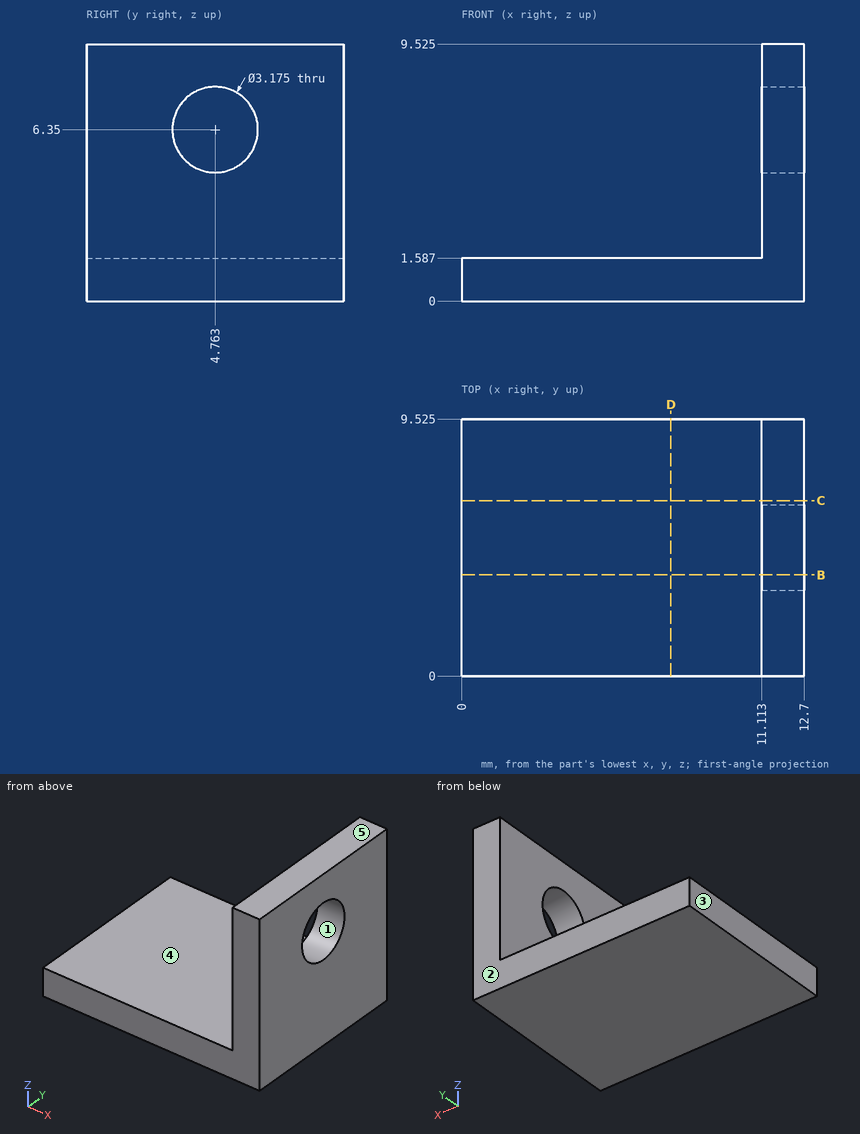
Check sheet for the drawn part. Datum: minimum x, y, z corner. Units: mm. A direction names the side the tool comes from. Round coordinates to 2 decimals unless told otherwise and drop trailing zeros. Write each loop counter-clockwise with the first axis right and the second up, starting at its lowest first coordinate (ties: lowest second). Pieces come first, ordered by that corner, then holes. Notation, with made-up numbers: (24.25, 74) -> (73.25, 74) arc R10 ccw to (73.25, 80) -> close; hole circle Ø7 at (-19, 16). An arc over 180 degrees is marked (long way). Write each question's results on one line, items separated by ' | '.
Q1. Draft check along Y on the marked faces 1, 2 and 3. Enter one of: released by +Y, released by -Y, zero draft, split by the parting line, or undercut.
Derived:
face 1: undercut | face 2: released by +Y | face 3: zero draft
Q2. Sectioned sample at C-C, the plane y = 6.5. Record the boundary of the cut face in (x, z) (1 decimal).
Derived:
outline: (0, 0) -> (12.7, 0) -> (12.7, 9.5) -> (11.1, 9.5) -> (11.1, 1.6) -> (0, 1.6) -> close
Q3. Thickness scan on probe 1 along Z at (x, y) = (3.5, 5); probe 2 along X at (y, z) = (1, 8.5); probe 3 along Z at (x, y) = (11.5, 3.75) (1 decimal). Record the ranges inside material, lowest first.
Derived:
probe 1: z = 0 to 1.59 | probe 2: x = 11.11 to 12.7 | probe 3: z = 0 to 5.1, 7.6 to 9.5
Q4. Sectioned sample at D-D, the plane x = 7.75. Record the boundary of the cut face in (y, z) (1 decimal), and give its area (3 significant figures).
Derived:
outline: (0, 0) -> (9.5, 0) -> (9.5, 1.6) -> (0, 1.6) -> close | area: 15.1 mm²
Q5. Access from +Z, -Z, +X, -X, +Y, -Y to the whole of each face (thin tool, end or side, straight path). Record for the marked faces 4 and 5.
Derived:
face 4: +Z, -X, +Y, -Y | face 5: +Z, +X, -X, +Y, -Y
Q6. Go/stop test with flat-tipped pins: pin 1 Ø3 at (x, y) = (7.5, 3) entering from +Z; pin 2 Ø1.5 at (x, z) = (9, 8) entering from +Y; pin 3 Ø2.5 at (y, z) = (5.5, 4) entering from -X; pin 4 Ø3 at (y, z) = (3.5, 6) entering from +X. Record where each tip stops, or that it passes through.
Derived:
pin 1: stops at z = 1.59 | pin 2: passes through | pin 3: stops at x = 11.11 | pin 4: stops at x = 12.7
Q7. Sectioned sample at B-B, the plane y = 3.75. Record the boundary of the cut face in (x, z) (1 decimal).
Derived:
outline: (0, 0) -> (12.7, 0) -> (12.7, 5.1) -> (11.1, 5.1) -> (11.1, 1.6) -> (0, 1.6) -> close; (11.1, 7.6) -> (12.7, 7.6) -> (12.7, 9.5) -> (11.1, 9.5) -> close
